from build123d import *

# Parameters (mm, degrees)
SKETCH1_W           = 43.63
SKETCH1_H           = 43.05
BOSS_EXTRUDE1_DEPTH = 1.13
SKETCH2_W           = 40.04
SKETCH2_H           = 34.12
BOSS_EXTRUDE2_DEPTH = 4
SKETCH4_W           = 36.91
SKETCH4_H           = 26.07
CUT_EXTRUDE1_DEPTH  = 1
FILLET1_R           = 3
SKETCH5_W           = 21
SKETCH5_H           = 9
BOSS_EXTRUDE3_DEPTH = 10
SKETCH6_W           = 8
SKETCH6_H           = 43.05
BOSS_EXTRUDE4_DEPTH = 2.2


with BuildPart() as part:
    # Sketch1 → Boss-Extrude1 (new body)
    with BuildSketch(Plane(origin=(0, 0, 0), x_dir=(1, 0, 0), z_dir=(0, 1, 0))):
        Rectangle(SKETCH1_W, SKETCH1_H)
    extrude(amount=BOSS_EXTRUDE1_DEPTH)

    # Sketch2 → Boss-Extrude2 (add)
    with BuildSketch(Plane(origin=(0, 1.13, 0), x_dir=(1, 0, 0), z_dir=(0, 1, 0))):
        with Locations((-0.205, 0.865)):
            Rectangle(SKETCH2_W, SKETCH2_H)
    extrude(amount=BOSS_EXTRUDE2_DEPTH)

    # Sketch4 → Cut-Extrude1 (cut)
    with BuildSketch(Plane(origin=(0, 5.13, 0), x_dir=(1, 0, 0), z_dir=(0, 1, 0))):
        with Locations((-0.15, -1.76)):
            Rectangle(SKETCH4_W, SKETCH4_H)
    extrude(amount=-CUT_EXTRUDE1_DEPTH, mode=Mode.SUBTRACT)

    # Fillet1
    fillet1_edges = [part.edges().sort_by_distance(p)[0] for p in [
        (-18.605, 4.63, 14.795),
        (-18.605, 4.63, -11.275),
        (18.305, 4.63, -11.275),
        (18.305, 4.63, 14.795),
    ]]
    fillet(fillet1_edges, radius=FILLET1_R)

    # Sketch5 → Boss-Extrude3 (add)
    with BuildSketch(Plane.XZ):
        with Locations((0, -17.025)):
            Rectangle(SKETCH5_W, SKETCH5_H)
    extrude(amount=BOSS_EXTRUDE3_DEPTH)

    # Sketch6 → Boss-Extrude4 (add)
    with BuildSketch(Plane.XZ):
        with Locations((17.815, 0)):
            Rectangle(SKETCH6_W, SKETCH6_H)
        with Locations((-17.815, 0)):
            Rectangle(SKETCH6_W, SKETCH6_H)
    extrude(amount=BOSS_EXTRUDE4_DEPTH)


solid = part.part
Source: CAD feature listing. Evaluate the final solid. Frame: model axes, mm. A direction names the side the tool comes from. Give positions to 0.01 mm unless a question says otherwise; leave off trailing zeros. Order: outer loops, then holes, each group sorted by start corner. A loop starts at its lowest first (then second) coordinate and runs counter-clockwise, first axis right, second up. Notation, with made-up numbers: (10, 44.25) -> (55, 44.25) arc R10 ccw to (55, 57.25) -> close; hole circle Ø9 at (65, 7.25). An arc over 180 degrees is marked (long way). Write item = value, one per line.
Q1. Set-up query: faces 1 (the face through (-0.4, 4.6, -11.275)), 2 (the face through (0, 3, -17.925)), 3 (the face through (19.815, 3, -1)), 4 (the face through (0, 3, 16.195)), 5 (the face through (-10.5, -5, -17)). Return all of +Z, -Z, +X, -X, +Y, -Y with unobstructed straight access to the full face (end or side cutting, diameter ignored); none if empty.
Data:
face_1 = +Y
face_2 = -Z, +X, -X, +Y
face_3 = +Z, -Z, +X, +Y
face_4 = +Z, +X, -X, +Y
face_5 = +Z, -Z, -Y
Q2. Cut plane A-A, the plane x = 5.5. Output: boundary loops of the cut face in (y, z) (3 decimals).
Data:
outline = (-10, -21.525) -> (1.13, -21.525) -> (1.13, -17.925) -> (5.13, -17.925) -> (5.13, -11.275) -> (4.13, -11.275) -> (4.13, 14.795) -> (5.13, 14.795) -> (5.13, 16.195) -> (1.13, 16.195) -> (1.13, 21.525) -> (0, 21.525) -> (0, -12.525) -> (-10, -12.525) -> close
Q3. Cut plane C-C, the plane y = -4.75. Output: boundary loops of the cut face in (x, z) (3 decimals).
Data:
outline = (-10.5, -21.525) -> (10.5, -21.525) -> (10.5, -12.525) -> (-10.5, -12.525) -> close
Q4. Cut plane D-D, the plane x = 14.5. Output: boundary loops of the cut face in (y, z) (3 decimals).
Data:
outline = (-2.2, -21.525) -> (1.13, -21.525) -> (1.13, -17.925) -> (5.13, -17.925) -> (5.13, -11.275) -> (4.13, -11.275) -> (4.13, 14.795) -> (5.13, 14.795) -> (5.13, 16.195) -> (1.13, 16.195) -> (1.13, 21.525) -> (-2.2, 21.525) -> close
Q5. Material intervals for line 1 (X direction, y = -1, z = -13) (3 decimals); line 2 (X direction, y = -1.25, z = 11.5) (3 decimals); line 3 (X direction, y = 4.25, z = 11.5) (3 decimals), sorted ascending. Write a range as from..to.
Data:
line_1 = -21.815..-13.815, -10.5..10.5, 13.815..21.815
line_2 = -21.815..-13.815, 13.815..21.815
line_3 = -20.225..-18.605, 18.305..19.815
Q6. Pull-direction query (X, two-part tool) for faces 6 (the face through (18, -2.2, 0)), 7 (the face through (0, 0, 4)), 8 (the face through (-20.225, 3, -1)); classes: released by +X, released by -X, zero draft, split by the parting line, or undercut.
Data:
face_6 = zero draft
face_7 = undercut
face_8 = released by -X
Q7. Pin query (flat end, axial travel): pin 1 (2.5 mm diameter, centred on y = -7, z = -17.5, fed in from +X); pin 2 (5 mm diameter, centred on x = -0.5, y = -5, fed in from +Z) (3 decimals); pin 3 (1.2 mm diameter, centred on x = 4.5, y = 3.5, fed in from +Z) (3 decimals). Return the tip coordinate at first contact, or that it passes through.
Data:
pin_1 = 10.5
pin_2 = -12.525
pin_3 = 16.195
Q8. Cut plane B-B, the plane z = 19. Output: boundary loops of the cut face in (x, y) (3 decimals), and give its area (3 significant figures).
Data:
outline = (-21.815, -2.2) -> (-13.815, -2.2) -> (-13.815, 0) -> (13.815, 0) -> (13.815, -2.2) -> (21.815, -2.2) -> (21.815, 1.13) -> (-21.815, 1.13) -> close
area = 84.5 mm^2
